Verification items for the finished model (mm, model axes). A direction names the side the tool comes from. Give positions to 0.01 mm unless a question says otherwise; leave off trailing zeros. Loops run counter-clockwise (first coordinate to the right, second up) from the corner with the lowest first, then second, coordinate; pieces in that order, holes last. Notation, with made-up numbers: (2, 77.5) - (45, 77.5) arc R5 ccw to (45, 83.5) - close; hole circle Ø3 at (83, 5). An arc over 180 degrees is marked (long way). Use one line per item in the form item = value.
Autodesk Inventor part; units mm, degrees
ref_plane "Work Plane2" through (0, 59.8, 0) normal (0, 1, 0) x (1, 0, 0)
ref_plane "YZ Plane" through (0, 0, 0) normal (1, 0, 0) x (0, 1, 0)
ref_plane "XZ Plane" through (0, 0, 0) normal (0, 1, 0) x (-1, 0, 0)
sketch "Sketch1" plane through (0, 0, 0) normal (0, 1, 0) x (-1, 0, 0)
  line L0 (-50, 82.5) -> (50, 82.5)
  line L1 (50, 82.5) -> (50, -82.5)
  line L2 (50, -82.5) -> (-50, -82.5)
  line L3 (-50, -82.5) -> (-50, 82.5)
  line L4 (-50, 82.5) -> (50, -82.5) construction
  line L5 (50, 82.5) -> (-50, -82.5) construction
  line L6 (-60, 92.5) -> (60, 92.5)
  line L7 (60, 92.5) -> (60, -92.5)
  line L8 (60, -92.5) -> (-60, -92.5)
  line L9 (-60, -92.5) -> (-60, 92.5)
  line L10 (-60, 92.5) -> (60, -92.5) construction
  line L11 (60, 92.5) -> (-60, -92.5) construction
  point P0 (0, 0)
  dimension "d0" = 100
  dimension "d1" = 165
  dimension "d2" = 120
  dimension "d3" = 185
extrude "Extrusion1" add sketch "Sketch1" along normal blind 75
ref_plane "Work Plane2" through (0, 59.8, 0) normal (0, 1, 0) x (1, 0, 0)
sketch "Sketch3" plane through (0, 59.8, 0) normal (0, 1, 0) x (1, 0, 0)
  line L0 (50, 82.5) -> (50, -82.5)
  line L1 (50, 82.5) -> (20, 82.5)
  line L2 (-50, 82.5) -> (50, 82.5)
  line L3 (50, 82.5) -> (50, 52.5)
  line L4 (50, 52.5) -> (20, 82.5)
  line L5 (50, -82.5) -> (50, -52.5)
  line L6 (50, -52.5) -> (20, -82.5)
  line L7 (50, -82.5) -> (-50, -82.5)
  line L8 (20, -82.5) -> (50, -82.5)
  line L9 (0, 82.5) -> (0, -82.5)
  line L10 (-50, 82.5) -> (-50, -82.5)
  line L11 (-50, 82.5) -> (-20, 82.5)
  line L12 (-50, 52.5) -> (-20, 82.5)
  line L13 (-50, -52.5) -> (-20, -82.5)
  line L14 (-50, -82.5) -> (50, -82.5)
  point P0 (0, 0)
  point P1 (-20, 82.5)
  dimension "d9" = 30
  dimension "d10" = 30
  dimension "d20" = 30
  dimension "d50" = 30
extrude "Extrusion3" add sketch "Sketch3" against normal blind 4 contours L0 L4 L1 | L0 L7 L6 | L12 L10 L2 | L7 L10 L13
sketch "Sketch5" plane through (0, 59.8, 0) normal (0, 1, 0) x (1, 0, 0)
  circle A0 centre (40, 72.5) radius 1.3
  line L0 (50, 82.5) -> (50, -82.5)
  line L1 (50, 0) -> (-50, 0)
  line L2 (-50, -82.5) -> (-50, 82.5)
  line L3 (50, -82.5) -> (-50, -82.5)
  line L4 (0, -82.5) -> (0, 82.5)
  line L5 (-50, 82.5) -> (50, 82.5)
  line L6 (50, -82.5) -> (20, -82.5)
  line L7 (50, -82.5) -> (40, -82.5)
  line L8 (40, -82.5) -> (40, -72.5)
  line L9 (40, -72.5) -> (50, -72.5)
  line L10 (50, -72.5) -> (50, -82.5)
  circle A1 centre (40, -72.5) radius 1.3
  line L11 (-50, 52.5) -> (-50, 82.5)
  line L12 (-50, 82.5) -> (-40, 82.5)
  line L13 (-40, 82.5) -> (-40, 72.5)
  line L14 (-40, 72.5) -> (-50, 72.5)
  line L15 (-50, 72.5) -> (-50, 82.5)
  circle A2 centre (-40, 72.5) radius 1.3
  line L16 (-50, -82.5) -> (-40, -82.5)
  line L17 (-40, -82.5) -> (-40, -72.5)
  line L18 (-40, -72.5) -> (-50, -72.5)
  line L19 (-50, -72.5) -> (-50, -82.5)
  circle A3 centre (-40, -72.5) radius 1.3
  dimension "d17" = 2.6
  dimension "d21" = 10
  dimension "d22" = 10
  dimension "d23" = 2.6
  dimension "d24" = 10
  dimension "d25" = 10
  dimension "d26" = 2.6
  dimension "d27" = 10
  dimension "d28" = 10
  dimension "d29" = 2.6
  dimension "d48" = 10
  dimension "d49" = 10
extrude "Extrusion5" cut sketch "Sketch5" against normal blind 4 contours A0 | A1 L8 L9 | L9 L8 A1 | A2 L14 L13 | L13 L14 A2 | A3 L17 L18 | L18 L17 A3
sketch "Sketch10" plane through (0, 0, 0) normal (0, -1, 0) x (1, 0, 0)
  line L0 (55, -87.5) -> (-55, -87.5)
  line L1 (-55, -87.5) -> (-55, 87.5)
  line L2 (-55, 87.5) -> (55, 87.5)
  line L3 (55, 87.5) -> (55, -87.5)
  line L4 (55, -87.5) -> (-55, 87.5) construction
  line L5 (-55, -87.5) -> (55, 87.5) construction
  point P0 (0, 0)
  dimension "d38" = 110
  dimension "d39" = 175
extrude "Extrusion8" cut sketch "Sketch10" against normal blind 5
sketch "Sketch11" plane through (0, 0, 0) normal (0, -1, 0) x (1, 0, 0)
  line L0 (-55, -87.5) -> (-55, 87.5)
  line L1 (-60, -92.5) -> (-60, 92.5)
  circle A0 centre (-57.5, -90) radius 0.75
  line L2 (-60, -92.5) -> (-60, 92.5)
  circle A1 centre (-57.5, 90) radius 0.75
  line L3 (-60, 92.5) -> (60, 92.5)
  line L4 (55, 87.5) -> (55, -87.5)
  circle A2 centre (57.5, 90) radius 0.75
  line L5 (60, -92.5) -> (-60, -92.5)
  circle A3 centre (57.5, -90) radius 0.75
  point P0 (0, 0)
  dimension "d42" = 1.5
  dimension "d43" = 1.5
  dimension "d44" = 1.5
  dimension "d45" = 1.5
extrude "Extrusion9" cut sketch "Sketch11" against normal blind 5
sketch "Sketch12" plane through (0, 75, 0) normal (0, 1, 0) x (1, 0, 0)
  line L0 (-50.5, 83) -> (50.5, 83)
  line L1 (50.5, 83) -> (50.5, -83)
  line L2 (50.5, -83) -> (-50.5, -83)
  line L3 (-50.5, -83) -> (-50.5, 83)
  line L4 (-50.5, 83) -> (50.5, -83) construction
  line L5 (50.5, 83) -> (-50.5, -83) construction
  point P0 (0, 0)
  dimension "d51" = 101
  dimension "d52" = 166
extrude "Extrusion10" cut sketch "Sketch12" against normal blind 15.2
sketch "Sketch15" plane through (0, 59.8, 0) normal (0, 1, 0) x (1, 0, 0)
  line L0 (-20, 82.5) -> (-50, 52.5)
  line L1 (-50, 52.5) -> (-50, 67.5)
  line L2 (-50, 67.5) -> (-35, 67.5)
  line L3 (-35, 67.5) -> (-35, 52.5)
  line L4 (-35, 52.5) -> (-50, 52.5)
  line L5 (-50, 52.5) -> (-50, 67.5)
  point P0 (0, 0)
  dimension "d56" = 15
  dimension "d57" = 15
  dimension "d58" = 15
extrude "Extrusion11" cut sketch "Sketch15" against normal blind 4
sketch "Sketch16" plane through (-60, 0, 92.5) normal (0, 0, 1) x (1, 0, 0)
  line L0 (0, 0) -> (0, 75)
  line L1 (0, 0) -> (0, 15)
  line L2 (0, 15) -> (15, 15)
  line L3 (15, 15) -> (34.6, 15)
  line L4 (34.6, 15) -> (34.6, 28)
  line L5 (34.6, 28) -> (15, 28)
  line L6 (15, 28) -> (15, 15)
  point P0 (60, 0)
  dimension "d61" = 15
  dimension "d62" = 15
  dimension "d63" = 19.6
  dimension "d64" = 13
extrude "Extrusion12" cut sketch "Sketch16" against normal blind 10
sketch "Sketch18" plane through (20, 59.8, 82.5) normal (0, 0, -1) x (-1, 0, 0)
  line L0 (45.4, -44.8) -> (45.4, -31.8)
  line L1 (45.4, -31.8) -> (45.4, -28.8)
  line L2 (45.4, -28.8) -> (42.4, -28.8)
  line L3 (65, -31.8) -> (65, -44.8)
  line L4 (65, -44.8) -> (68, -44.8)
  line L5 (68, -44.8) -> (68, -47.8)
  line L6 (42.4, -28.8) -> (68, -28.8)
  line L7 (68, -28.8) -> (68, -47.8)
  line L8 (68, -47.8) -> (42.4, -47.8)
  line L9 (42.4, -47.8) -> (42.4, -28.8)
  point P0 (20, -59.8)
  dimension "d67" = 3
  dimension "d68" = 3
  dimension "d69" = 3
  dimension "d70" = 3
extrude "Extrusion13" cut sketch "Sketch18" against normal blind 7
sketch "Sketch19" plane through (-50, 55.8, 82.5) normal (1, 0, 0) x (0, 0, -1)
  line L0 (0, -50.8) -> (165, -50.8)
  circle A0 centre (114, -24.3) radius 10.75
  point P0 (82.5, -55.8)
  point P1 (114, -50.8)
  dimension "d73" = 51
  dimension "d74" = 26.5
  dimension "d75" = 21.5
extrude "Extrusion14" cut sketch "Sketch19" against normal blind 10
properties part number "Enclose Top" material "PC/ABS Plastic"
1. Section check B-B, the plane z = 55.5. Record the cut outline in (x, y).
Result set:
outline = (-60, 0) - (-55, 0) - (-55, 5) - (-50, 5) - (-50, 55.8) - (-47, 55.8) - (-47, 59.8) - (-50.5, 59.8) - (-50.5, 75) - (-60, 75) - close; (47, 55.8) - (50, 55.8) - (50, 5) - (55, 5) - (55, 0) - (60, 0) - (60, 75) - (50.5, 75) - (50.5, 59.8) - (47, 59.8) - close
2. Scan lines: probe 1 along X at (y, z) = (2, 90); probe 2 along X at (y, z) = (55.5, -36); probe 3 along Z at (x, y) = (36.5, 39). Record each from-to range of solid material in increasing order.
Result set:
probe_1 = -60 to -58.25, -56.75 to 56.75, 58.25 to 60
probe_2 = -60 to -50, 50 to 60
probe_3 = -92.5 to -82.5, 82.5 to 92.5
3. Section check D-D, the plane y = 34. Record the cut outline in (x, z), then the cut area to 3 significant figures.
Result set:
outline = (-60, -92.5) - (60, -92.5) - (60, 92.5) - (-60, 92.5) - (-60, -21.04) - (-50, -21.04) - (-50, 82.5) - (50, 82.5) - (50, -82.5) - (-50, -82.5) - (-50, -41.96) - (-60, -41.96) - close
area = 5,490 mm²
4. Draft check along X on faces 1 (the flat face through (35.2, 57.8, -67.3)), 2 (the cylindrical face through (-54.93, 34.729, -41.754)), 3 (the flat face through (50, 32, -1)). Enter one of: released by +X, released by -X, zero draft, split by the parting line, or undercut.
Result set:
face_1 = undercut
face_2 = zero draft
face_3 = undercut
5. Section check A-A, the plane x = -31.5. Record the cut outline in (y, z).
Result set:
outline = (0, -92.5) - (75, -92.5) - (75, -83) - (59.8, -83) - (59.8, -71) - (55.8, -71) - (55.8, -82.5) - (5, -82.5) - (5, -87.5) - (0, -87.5) - close; (0, 87.5) - (5, 87.5) - (5, 82.5) - (12, 82.5) - (12, 89.5) - (15, 89.5) - (15, 92.5) - (0, 92.5) - close; (28, 89.5) - (31, 89.5) - (31, 82.5) - (55.8, 82.5) - (55.8, 71) - (59.8, 71) - (59.8, 83) - (75, 83) - (75, 92.5) - (28, 92.5) - close
6. Section check C-C, the plane y = 45. Record the cut outline in (x, z).
Result set:
outline = (-60, -92.5) - (60, -92.5) - (60, 92.5) - (-60, 92.5) - close; hole (-50, -82.5) - (50, -82.5) - (50, 82.5) - (-50, 82.5) - close
7. Tool access check on faces 4 (the flat face through (50.5, 68, -1)), 5 (the flat face through (-27.6, 57.8, -74.9)), 6 (the flat face through (-35, 13, 89.5)), 7 (the flat face through (-39, 55.8, -75)). Record the directions out of +Z, -Z, +X, -X, +Y, -Y that give a thin tool (end or side, any length) a straight path to the whole face; none if there is none.
Result set:
face_4 = +Y
face_5 = +Y, -Y
face_6 = none
face_7 = -Y
8. Depth check by flat-ended pin: pin 1 Ø1 at (x, y) = (-35, 17) entering from +Z; pin 2 Ø6 at (x, z) = (32, 67.5) entering from -Y; pin 3 Ø13 at (y, z) = (31.5, -31.5) entering from -X. Enter the tip coordinate at first touch or a pass-through.
Result set:
pin_1 = -82.5
pin_2 = 55.8
pin_3 = 50
